Here's how the part is built. I have some questions about the finished solid (model axes, mm). A direction names the side the tool comes from. Give positions to 0.01 mm unless a question says otherwise; leave off trailing zeros. Loops run counter-clockwise (first coordinate to the right, second up) from the corner with the lowest first, then second, coordinate; pieces in that order, holes last. Notation, with made-up numbers: M 89.5,81 L 100.5,81 A13 cw 100.5,104 Z; hole C 35,-5.75 d7. An arc over 180 degrees is marked long. Answer as CSV lines item,"result". Start each with the question number.
Item 1: I want a section at B-B on x = 0. List the corners of the cut face in (y, z) for me, plus the area to 3 significant figures.
Item 2: For faces 4 (the flat face through (5, -2, 0)), 5 (the cylindrical face through (1.74, -12.4, 22.38)), 6 (the flat face through (0, -20, 20)), which set-ups out of +Z, -Z, +X, -X, +Y, -Y let a thin tool reach every point of the face, with its end or its side?
Item 3: I want a section at A-A on z = 0. List the corners of the cut face in (x, y) for me.
Item 4: Will these pins go through, and if not, where does the flat tip stop? P1, Ø4, axis at x = -2, y = -2.5, coming from the +Z side; P2, Ø2, axis at x = 5.5, y = -3.5, coming from the +Z side; P3, Ø2, axis at x = 5, y = -14.5, coming from the -Z side; P4, Ø10, axis at x = 10.5, z = 0.5, coming from the -Y side.
Item 5: If we mould it in two halves opening along X, with no side actions, what happens to faces 1 (the cylindrical face through (23.846, -2.479, 7.509)), 2 (the flat face through (-17, -20, -10)), 3 (the flat face through (0, -2, 5))? For each: released by +X, released by -X, zero draft, split by the parting line, or undercut.
Item 6: I want a section at C-C on y = -17.25. List the corners of the cut face in (x, z) for me, plus the area to 3 significant figures.
Item 7: If I drill on line 1 along Z through (x, y) = (0.5, -3) (3 decimals); line 2 along Y through (x, z) = (-0.5, -22.5); line 3 along X through (y, z) = (-13.5, -10.5), over which ranges is the centre line in solid material (lowest first)? Write a range as from..to.
from build123d import *

# Parameters (mm, degrees)
F0_R     = 3.2275405411
F1_DEPTH = 20
F0_R_2   = 25
F0_W     = 10
F0_H     = 10
F2_DEPTH = 5
F3_R     = 1


with BuildPart() as f1:
    # F0 (on Front) → F1 (new body)
    with BuildSketch(Plane.XZ):
        with Locations((17.0290375666, -9.8317194231)):
            Circle(F0_R)
    extrude(amount=F1_DEPTH)



with BuildPart() as f1b:
    # F0 (on Front) → F1, piece 2 (new body)
    with BuildSketch(Plane.XZ):
        with Locations((-17.0290375666, -9.8317194231)):
            Circle(F0_R)
    extrude(amount=F1_DEPTH)


with BuildPart() as f1c:
    # F0 (on Front) → F1, piece 3 (new body)
    with BuildSketch(Plane.XZ):
        with Locations((0, 19.6634388463)):
            Circle(F0_R)
    extrude(amount=F1_DEPTH)


with BuildPart() as f1_1:
    add(f1.part)

    add(f1b.part)  # F2 merges F1b

    add(f1c.part)  # F2 merges F1c
    # F0 (on Front) → F2 (join)
    with BuildSketch(Plane.XZ):
        Circle(F0_R_2)
        with Locations((-17.0290375666, -9.8317194231)):
            Circle(F0_R, mode=Mode.SUBTRACT)
        with Locations((17.0290375666, -9.8317194231)):
            Circle(F0_R, mode=Mode.SUBTRACT)
        Rectangle(F0_W, F0_H, mode=Mode.SUBTRACT)
        with Locations((0, 19.6634388463)):
            Circle(F0_R, mode=Mode.SUBTRACT)
    extrude(amount=F2_DEPTH)

    # F3
    f3_edges = [f1_1.edges().sort_by_distance(p)[0] for p in [
        (-25, 0, 0),
        (-25, -5, 0),
    ]]
    fillet(f3_edges, radius=F3_R)


solid = f1_1.part
Result:
1,outline,"M -20,16.44 L -5,16.44 L -5,5 L 0,5 L 0,24 A1 ccw -1,25 L -4,25 A1 ccw -5,24 L -5,22.89 L -20,22.89 Z; M -5,-24 A1 ccw -4,-25 L -1,-25 A1 ccw 0,-24 L 0,-5 L -5,-5 Z"
1,area,"296 mm^2"
2,face 4,"+Y, -Y"
2,face 5,"-Y"
2,face 6,"+Z, -Z, +X, -X, -Y"
3,outline,"M -25,-4 A1 ccw -24,-5 L -5,-5 L -5,0 L -24,0 A1 ccw -25,-1 Z; M 5,-5 L 24,-5 A1 ccw 25,-4 L 25,-1 A1 ccw 24,0 L 5,0 Z"
4,P1,"z = 25"
4,P2,"z = 24.59"
4,P3,"through"
4,P4,"y = -5"
5,face 1,"split by the parting line"
5,face 2,"zero draft"
5,face 3,"undercut"
6,outline,"C -17.03,-9.83 d6.46; C 0,19.66 d6.46; C 17.03,-9.83 d6.46"
6,area,"98.2 mm^2"
7,line 1,"-24.995..-5, 5..24.995"
7,line 2,"-5..0"
7,line 3,"-20.19..-13.87, 13.87..20.19"
